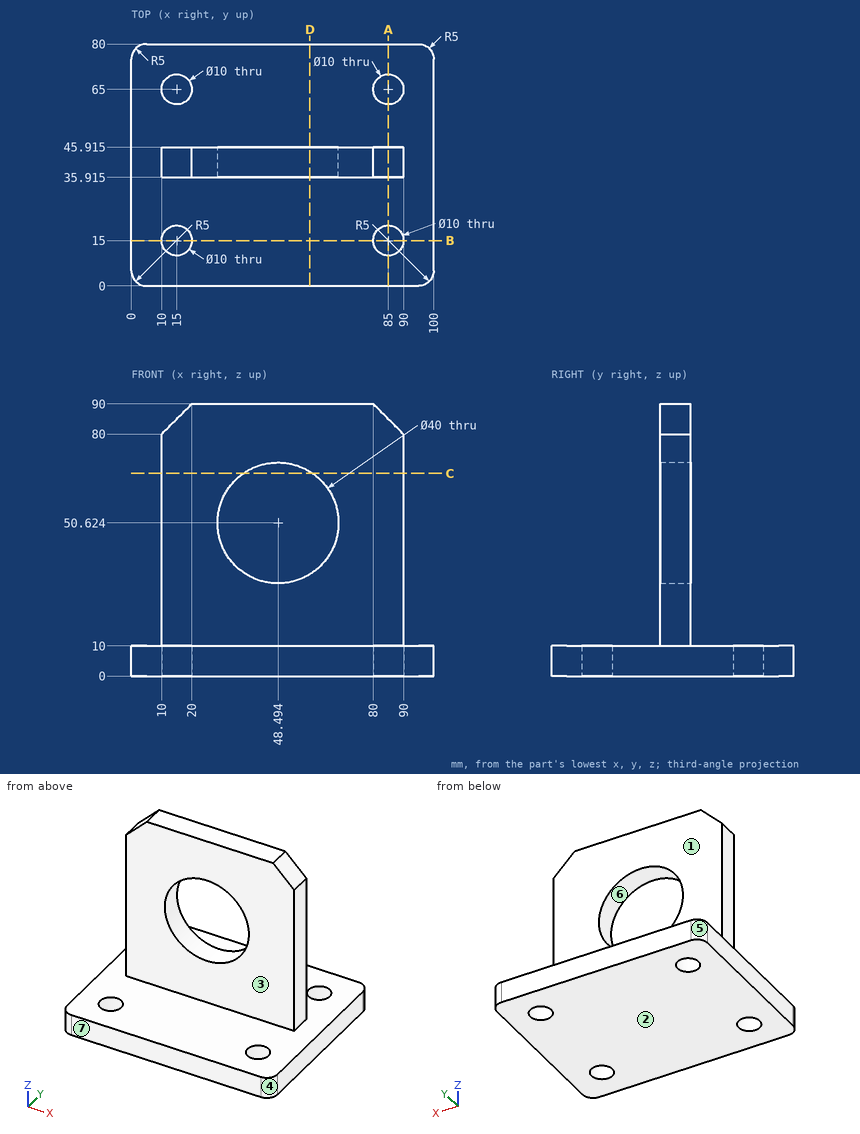
Geometry: see drawing. Coordinates: mm, zero at the bounding-box minimum. A direction names the side the tool comes from. Coordinates: 2 decimals unless noted, no trailing zeros. Loops run counter-clockwise (first coordinate to the right, second up) from the corner with the lowest first, then second, coordinate; pieces in that order, holes last. Notation, with made-up numbers: (88.5, 77.5) -> (138.5, 77.5) arc R28 ccw to (138.5, 101.5) -> close; hole circle Ø4 at (-4.75, 57). An arc over 180 degrees is marked (long way). Write item = value, one per line. Start each with the question number.
Item 1: Reachability of the marked faces 1, 2 and 3 from +Z, -Z, +X, -X, +Y, -Y: full face, straight path, thin tool, end or side. Return the list, or none.
Item 2: Mould query, pull axis X, two halves, no side actions, for the marked faces 4, 5, 6 and 7. Classes: pulls with the +X half, pulls with the -X half, needs draft (parallel to the pull), parting line crosses it, or undercut.
Item 3: Cut plane B-B, the plane y = 15. Return loops of the section in (x, z).
Item 4: Cut plane D-D, the plane x = 59. Return loops of the section in (y, z) (1 decimal).
Item 5: Cut plane A-A, the plane x = 85. Return loops of the section in (y, z) (1 decimal).
Item 6: Cut plane C-C, the plane z = 67. Return loops of the section in (x, y) (1 decimal), plus the area to 3 significant figures.
Item 7: First-contact query: P1, Ø11.5, axis at x = 15, y = 15, coming from the -Z side; P2, Ø24, axis at x = 53.5, y = 20, coming from the +Z side; P3, Ø3, axis at y = 40.5, z = 35, coming from the -X side; P4, Ø5, axis at y = 40, z = 35.5, coming from the +X side. Flat tips, straight axial feed; report the tip coordinate or a pass-through.
Item 8: Material intervals for line 1 (Y direction, x = 85, z = 3.75); line 2 (Z direction, x = 7, y = 12); line 3 (Y direction, x = 20, z = 44.5) (1 decimal), sorted ascending.
Ans:
q1.face_1 = +Z, +X, -X, +Y
q1.face_2 = -Z, +X, -X, +Y, -Y
q1.face_3 = +Z, +X, -X, -Y
q2.face_4 = pulls with the +X half
q2.face_5 = pulls with the -X half
q2.face_6 = undercut
q2.face_7 = needs draft
q3.outline = (0, 0) -> (10, 0) -> (10, 10) -> (0, 10) -> close; (20, 0) -> (80, 0) -> (80, 10) -> (20, 10) -> close; (90, 0) -> (100, 0) -> (100, 10) -> (90, 10) -> close
q4.outline = (0, 0) -> (80, 0) -> (80, 10) -> (45.9, 10) -> (45.9, 33.6) -> (35.9, 33.6) -> (35.9, 10) -> (0, 10) -> close; (35.9, 67.6) -> (45.9, 67.6) -> (45.9, 90) -> (35.9, 90) -> close
q5.outline = (0, 0) -> (10, 0) -> (10, 10) -> (0, 10) -> close; (20, 0) -> (60, 0) -> (60, 10) -> (45.9, 10) -> (45.9, 85) -> (35.9, 85) -> (35.9, 10) -> (20, 10) -> close; (70, 0) -> (80, 0) -> (80, 10) -> (70, 10) -> close
q6.outline = (10, 35.9) -> (37, 35.9) -> (37, 45.9) -> (10, 45.9) -> close; (60, 35.9) -> (90, 35.9) -> (90, 45.9) -> (60, 45.9) -> close
q6.area = 570 mm²
q7.P1 = 0
q7.P2 = 10
q7.P3 = 10
q7.P4 = 90
q8.line_1 = 0 to 10, 20 to 60, 70 to 80
q8.line_2 = 0 to 10
q8.line_3 = 35.9 to 45.9
